Verification items for this drawing (mm, ordinates from the low corner). A direction names the side the tool comes from. Coordinates: 2 decimals unless noted, no trailing zeros. Write each loop counter-clockwise with the first axis right and the second up, starting at its lowest first coordinate (ties: lowest second). Pieces come first, ordered by that corner, then holes. Notation, with made-up numbers: (-20.5, -24) -> (28.5, -24) arc R8 cw to (28.5, -17) -> close; hole circle Ø7 at (47, -0.75). An arc over 180 degrees is marked (long way). Use CSV: the item, a comma, the result in double quotes.
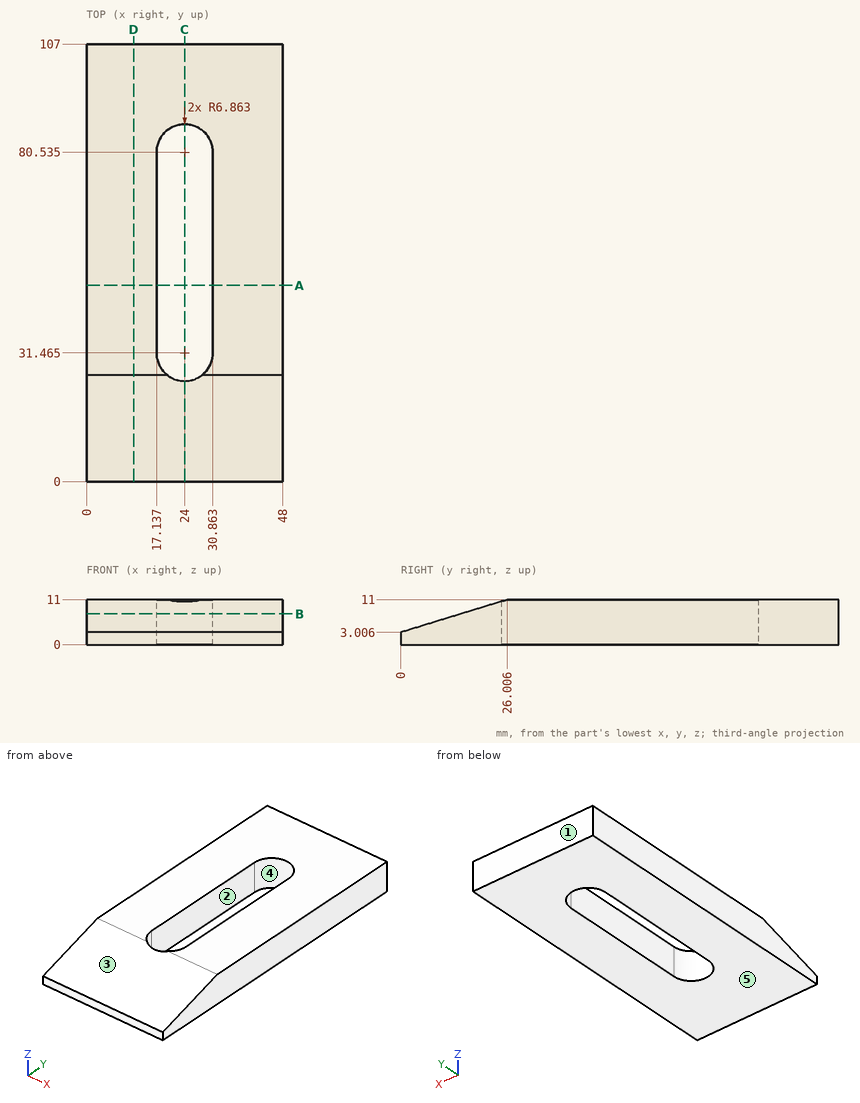
1) Cross-section at C-C (x = 24). Record the boundary of the cut face in (y, z), plus the area to 3 significant figures.
Return value:
outline,"(0, 0) -> (24.6, 0) -> (24.6, 10.57) -> (0, 3.01) -> close; (87.4, 0) -> (107, 0) -> (107, 11) -> (87.4, 11) -> close"
area,"383 mm2"
2) Mould release check, pull along Y, two halves, no side actions. Record for the marked faces 3, 4 and 5: released by +Y, released by -Y, zero draft, split by the parting line, or undercut.
Return value:
face 3,"released by -Y"
face 4,"undercut"
face 5,"zero draft"
3) Set-up check for the marked faces 1 and 2: record each of +Z, -Z, +X, -X, +Y, -Y from which the full face is reachable in a straight line by a thin tool's end or side.
Return value:
face 1,"+Z, -Z, +X, -X, +Y"
face 2,"+Z, -Z"
4) Cross-section at D-D (x = 11.5). Record the boundary of the cut face in (y, z).
Return value:
outline,"(0, 0) -> (107, 0) -> (107, 11) -> (26.01, 11) -> (0, 3.01) -> close"
5) Cross-section at B-B (z = 7.5). Record the boundary of the cut face in (x, y) (1 decimal), plus the area to 3 significant figures.
Return value:
outline,"(0, 14.6) -> (48, 14.6) -> (48, 107) -> (0, 107) -> close; hole (17.1, 31.5) arc R6.9 ccw to (30.9, 31.5) -> (30.9, 80.5) arc R6.9 ccw to (17.1, 80.5) -> close"
area,"3,610 mm2"
6) Scan lines: L1, parallel to X at y = 39, z = 10; L2, parallel to X at y = 29.5, z = 4.5 (1 decimal); L3, parallel to Y at x = 20, z = 0.75. Record each from-to range of solid material in increasing order.
Return value:
L1,"0 to 17.14, 30.86 to 48"
L2,"0 to 17.4, 30.6 to 48"
L3,"0 to 25.89, 86.11 to 107"
7) Cross-section at A-A (y = 48). Record the boundary of the cut face in (x, z).
Return value:
outline,"(0, 0) -> (17.14, 0) -> (17.14, 11) -> (0, 11) -> close; (30.86, 0) -> (48, 0) -> (48, 11) -> (30.86, 11) -> close"
